```python
from build123d import *

# Parameters (mm, degrees)
ESBO_O1_R                  = 2
RESSALTO_EXTRUS_O1_DEPTH   = 33.5
CORTE_EXTRUS_O3_START      = -5
CORTE_EXTRUS_O3_DEPTH      = 23.196699141
CORTE_EXTRUS_O4_DEPTH      = 47.084705336
CORTE_EXTRUS_O4_DEPTH_BACK = 47.084705336
ESBO_O4_W                  = 59
ESBO_O4_H                  = 6.231727984
CORTE_EXTRUS_O5_DEPTH      = 44.128413036
RESSALTO_EXTRUS_O3_START   = -29.398953743
RESSALTO_EXTRUS_O3_DEPTH   = 58.797908802
ESBO_O6_W                  = 59
ESBO_O6_H                  = 4.4
RESSALTO_EXTRUS_O4_DEPTH   = 0.5
CORTE_EXTRUS_O6_DEPTH      = 71.593909086
FILETE1_R                  = 2


# Read off the part's stored shape, not the designer's step: Corte-extrusão3, Ressalto-extrusão3
with BuildPart() as part:
    # Esboço1 → Ressalto-extrusão1 (new, symmetric)
    with BuildSketch(Plane(origin=(0, 0, 0), x_dir=(0, 0, -1), z_dir=(1, 0, 0))):
        with BuildLine():
            Line((-5, 0), (-5, -3))
            Line((-5, -3), (-23.5, -21.5))
            Line((-23.5, -21.5), (-11.6, -21.5))
            Line((-11.6, -21.5), (-11.6, -19.6))
            Line((-11.6, -19.6), (5, -3))
            Line((5, -3), (5, 0))
            ThreePointArc((5, 0), (0, 5), (-5, 0))
        make_face()
        Circle(ESBO_O1_R, mode=Mode.SUBTRACT)
    extrude(amount=RESSALTO_EXTRUS_O1_DEPTH, both=True)

    # Corte-extrusão3 outline → Corte-extrusão3 (cut)
    with BuildSketch(Plane.XY.offset(CORTE_EXTRUS_O3_START)):
        with BuildLine():
            Line((-25.5, -16.196699141), (25.5, -16.196699141))
            add(Edge.make_bspline(
                [(25.5, -16.196699141), (29.5, -16.196699141), (29.5, -13.368272016)],
                knots=[3.141592654, 3.141592654, 3.141592654, 4.71238898, 4.71238898, 4.71238898], degree=2, weights=[1, 0.707106781, 1]))
            Line((29.5, -13.368272016), (29.5, 6))
            Line((29.5, 6), (-29.5, 6))
            Line((-29.5, 6), (-29.5, -13.368272016))
            add(Edge.make_bspline(
                [(-29.5, -13.368272016), (-29.5, -16.196699141), (-25.5, -16.196699141)],
                knots=[4.71238898, 4.71238898, 4.71238898, 6.283185307, 6.283185307, 6.283185307], degree=2, weights=[1, 0.707106781, 1]))
        make_face()
    extrude(amount=CORTE_EXTRUS_O3_DEPTH, mode=Mode.SUBTRACT)

    # Esboço4 → Corte-extrusão4 (cut, two sides: drawn at the far end of the back side and taken through both)
    with BuildSketch(Plane(origin=(0, -16.196699141, 0), x_dir=(1, 0, 0), z_dir=(0, 1, 0)).offset(-CORTE_EXTRUS_O4_DEPTH_BACK)):
        with Locations((0, -8.484136008)):
            Rectangle(ESBO_O4_W, ESBO_O4_H)
    extrude(amount=CORTE_EXTRUS_O4_DEPTH + CORTE_EXTRUS_O4_DEPTH_BACK, mode=Mode.SUBTRACT)

    # Esboço5 → Corte-extrusão5 (cut, through all)
    with BuildSketch(Plane(origin=(0, 0, 11.6), x_dir=(-1, 0, 0), z_dir=(0, 0, -1))):
        with BuildLine():
            Line((29.398953619, -14), (29.5, -14))
            Line((29.5, -14), (29.5, -13.368272016))
            add(Edge.make_bspline(
                [(29.398953619, -14), (29.423863493, -13.923129609), (29.445428126, -13.845331175), (29.463538827, -13.766752142), (29.478105641, -13.68755334), (29.489060697, -13.607909452), (29.49636233, -13.528009486), (29.5, -13.448057281), (29.5, -13.368272016)],
                knots=[0.878269136, 0.878269136, 0.878269136, 0.878269136, 0.878269136, 0.878269136, 0.878269136, 0.878269136, 0.878269136, 1, 1, 1, 1, 1, 1, 1, 1, 1], degree=8))
        make_face()
        with BuildLine():
            Line((-29.5, -14), (-29.39895364, -14))
            add(Edge.make_bspline(
                [(-29.5, -13.368272016), (-29.5, -13.38237401), (-29.499886362, -13.396480452), (-29.499658961, -13.410590284), (-29.499317701, -13.424702445), (-29.498862515, -13.438815874), (-29.498293368, -13.452929509), (-29.497610253, -13.467042285), (-29.493100454, -13.546882135), (-29.48691474, -13.612580226), (-29.478257806, -13.678128457), (-29.467147216, -13.743415855), (-29.45361408, -13.808339118), (-29.437701062, -13.872802316), (-29.419460639, -13.936716614), (-29.39895364, -14)],
                knots=[0, 0, 0, 0, 0, 0, 0, 0, 0, 0.021519038, 0.021519038, 0.021519038, 0.021519038, 0.021519038, 0.021519038, 0.021519038, 0.121755683, 0.121755683, 0.121755683, 0.121755683, 0.121755683, 0.121755683, 0.121755683, 0.121755683, 0.121755683], degree=8))
            Line((-29.5, -13.368272016), (-29.5, -14))
        make_face()
    extrude(amount=-CORTE_EXTRUS_O5_DEPTH, mode=Mode.SUBTRACT)

    # Ressalto-extrusão3 outline → Ressalto-extrusão3 (add)
    with BuildSketch(Plane.YZ.offset(RESSALTO_EXTRUS_O3_START)):
        Polygon((-14, 16), (-16.196699141, 18.196699141), (-16.196699141, 11.6), (-14, 11.6), align=None)
    extrude(amount=RESSALTO_EXTRUS_O3_DEPTH)

    # Esboço6 → Ressalto-extrusão4 (add)
    with BuildSketch(Plane(origin=(0, -14, 0), x_dir=(1, 0, 0), z_dir=(0, 1, 0))):
        with Locations((0, -13.8)):
            Rectangle(ESBO_O6_W, ESBO_O6_H)
    extrude(amount=RESSALTO_EXTRUS_O4_DEPTH)

    # Esboço7 → Corte-extrusão6 (cut, through all)
    with BuildSketch(Plane.ZY.offset(29.5)):
        Polygon((16, -13.5), (15.5, -13.5), (16, -14), align=None)
    extrude(amount=-CORTE_EXTRUS_O6_DEPTH, mode=Mode.SUBTRACT)

    # Filete1
    filete1_edges = [part.edges().sort_by_distance(p)[0] for p in [
        (29.5, -13.5, 13.55),
        (-29.5, -13.5, 13.55),
    ]]
    fillet(filete1_edges, radius=FILETE1_R)


solid = part.part
```
Design review of the part built by this model. Coordinates are the model's own, in mm. A direction names the side the tool comes from. Coordinates: 2 decimals unless noted, no trailing zeros. Loops run counter-clockwise (first coordinate to the right, second up) from the corner with the lowest first, then second, coordinate; pieces in that order, holes last. Notation, with made-up numbers: (20.25, 73.5) -> (60.25, 73.5) arc R21 ccw to (60.25, 97.5) -> close; hole circle Ø11 at (35.5, 8). An arc over 180 degrees is marked (long way). Answer as a JSON object with one key per item and string values.
Q1. Take a section at D-D on x = 1.5. Give the boundary of the cut face in (y, z).
Answer block:
{"outline": "(-21.5, 11.6) -> (-13.5, 11.6) -> (-13.5, 15.5) -> (-21.5, 23.5) -> close"}
Q2. Clearance check with flat-ended pins moving along their axes: pin 1 Ø3.5 at (x, y) = (-32, -1.5) entering from +Z; pin 2 Ø8 at (x, y) = (13.5, -15) entering from -Z; pin 3 Ø8 at (x, z) = (-9.5, 14) entering from +Y. State where each tip first meets the part, or that it passes through.
Answer block:
{"pin 1": "stops at z = 5.25", "pin 2": "stops at z = 11.6", "pin 3": "stops at y = -13.5"}
Q3. To check wall thickness, follow L1, parallel to X at y = -14.5, z = 9; L2, parallel to Y at x = 11.5, z = 13; L3, parallel to Y at x = -32.5, z = 0. State the ranges of each line that lie inside material, in increasing order.
Answer block:
{"L1": "x = -33.5 to -29.5, 29.5 to 33.5", "L2": "y = -21.5 to -13.5", "L3": "y = -8 to -2, 2 to 5"}
Q4. Take a section at A-A on z = 0. Give the boundary of the cut face in (x, y).
Answer block:
{"outline": "(-33.5, -8) -> (-29.5, -8) -> (-29.5, -2) -> (-33.5, -2) -> close; (-33.5, 2) -> (-29.5, 2) -> (-29.5, 5) -> (-33.5, 5) -> close; (29.5, -8) -> (33.5, -8) -> (33.5, -2) -> (29.5, -2) -> close; (29.5, 2) -> (33.5, 2) -> (33.5, 5) -> (29.5, 5) -> close"}
Q5. The part is to be moulded in two halves that separate along X. For faces 4 (the flat face through (32, -1, 5)), 5 (the flat face through (-33.5, -10, 7)), 6 (the flat face through (0, -13.5, 14)), say which applies: +X half, -X half, draft (parallel to the pull), parting line (faces both ways), or undercut.
Answer block:
{"face 4": "draft", "face 5": "-X half", "face 6": "undercut"}
Q6. Tool access review of faces 1 (the cylindrical face through (32, 5, 0)), 2 (the flat face through (-31, -1, 5)), 3 (the cylindrical face through (28.93, -12.9, 13.09)): name each direction out of +Z, -Z, +X, -X, +Y, -Y from which nothing blocks a thin tool from reaching the whole face with its end or side.
Answer block:
{"face 1": "+X, -X, +Y", "face 2": "+Z, +X, -X, +Y", "face 3": "+Z, -Z, +Y"}
Q7. Take a section at B-B on z = -3.5. Give the boundary of the cut face in (x, y), plus the area to 3 significant figures.
Answer block:
{"outline": "(-33.5, -4.5) -> (-29.5, -4.5) -> (-29.5, 3.57) -> (-33.5, 3.57) -> close; (29.5, -4.5) -> (33.5, -4.5) -> (33.5, 3.57) -> (29.5, 3.57) -> close", "area": "64.6 mm^2"}
Q8. Take a section at C-C on z = 12.25. Give the boundary of the cut face in (x, y), plus the area to 3 significant figures.
Answer block:
{"outline": "(-33.5, -21.5) -> (33.5, -21.5) -> (33.5, -10.25) -> (29.5, -10.25) -> (29.5, -11.5) arc R2 cw to (27.5, -13.5) -> (-27.5, -13.5) arc R2 cw to (-29.5, -11.5) -> (-29.5, -10.25) -> (-33.5, -10.25) -> close", "area": "564 mm^2"}
